```python
from build123d import *

# Parameters (mm, degrees)
SKETCH1_W           = 55.65
SKETCH1_H           = 70.9
BOSS_EXTRUDE1_DEPTH = 5
SKETCH3_W           = 53.15
SKETCH3_H           = 68.4
CUT_EXTRUDE1_DEPTH  = 3
SKETCH2_R           = 2.5
CUT_EXTRUDE2_DEPTH  = 6


with BuildPart() as part:
    # Sketch1 → Boss-Extrude1 (new body)
    with BuildSketch(Plane.XY):
        Rectangle(SKETCH1_W, SKETCH1_H)
    extrude(amount=BOSS_EXTRUDE1_DEPTH)

    # Sketch3 → Cut-Extrude1 (cut)
    with BuildSketch(Plane(origin=(0, 0, 0), x_dir=(-1, 0, 0), z_dir=(0, 0, -1))):
        Rectangle(SKETCH3_W, SKETCH3_H)
    extrude(amount=-CUT_EXTRUDE1_DEPTH, mode=Mode.SUBTRACT)

    # Sketch2 → Cut-Extrude2 (cut, through all)
    with BuildSketch(Plane(origin=(0, 0, 0), x_dir=(-1, 0, 0), z_dir=(0, 0, -1))):
        with Locations((-8.973470341, 31.308167243)):
            Circle(SKETCH2_R)
        with Locations((-23.973470341, -18.491832757)):
            Circle(SKETCH2_R)
        with Locations((23.676529659, -20.991832757)):
            Circle(SKETCH2_R)
        with Locations((19.676529659, 31.308167243)):
            Circle(SKETCH2_R)
    extrude(amount=-CUT_EXTRUDE2_DEPTH, mode=Mode.SUBTRACT)


solid = part.part
```
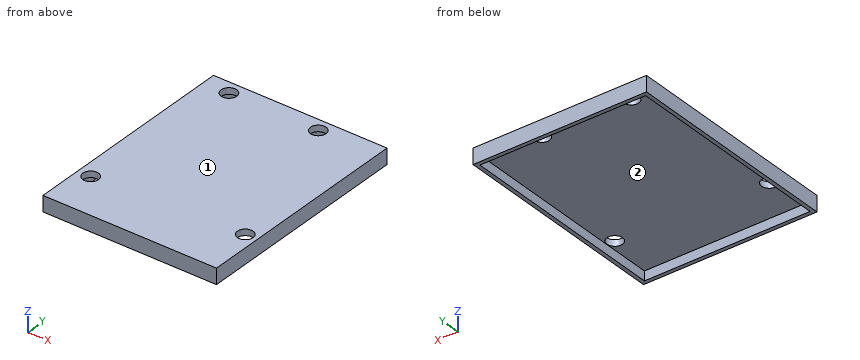
Verification items for the finished model (mm, model axes). Face numbers are marked on the shaded views. Round coordinates to 2 decimals unless told otherwise and drop trailing zeros. Write each loop counter-clockwise with the first axis right and the second up, starting at its lowest first coordinate (ties: lowest second). Pieces come first, ordered by that corner, then holes.
1. Section check D-D on x = -7.5. Enter the section's corners in (y, z).
2. Scan lines: L1, parallel to X at y = 3, z = 2.9 (3 decimals); L2, parallel to Y at x = 10, z = 1.25; L3, parallel to Y at x = 9, z = 3.4. Record each from-to range of solid material in increasing order.
3. Draft check along X on the marked faces 1 and 2. Enter one of: +X half, -X half, draft (parallel to the pull), parting line (faces both ways), or undercut.
4. Section check C-C on x = 9. Enter the section's corners in (y, z), plus the area to 3 significant figures.
5. Section check A-A on z = 1.9. Enter the section's corners in (x, y) (3 decimals).
6. Section check B-B on y = -2.5. Enter the section's corners in (x, z) (3 decimals).
7. Gauge pin test, flat end, axial feed: P1, Ø1.5, axis at x = 20.5, y = 8, coming from the -Z side. Record the tip position at first contact, or that the pin passes through.
Answer:
1. outline: (-35.45, 0) - (-34.2, 0) - (-34.2, 3) - (34.2, 3) - (34.2, 0) - (35.45, 0) - (35.45, 5) - (-35.45, 5) - close
2. L1: x = -27.825 to -26.575, 26.575 to 27.825
2. L2: y = -35.45 to -34.2, 34.2 to 35.45
2. L3: y = -35.45 to 28.81, 33.81 to 35.45
3. face 1: draft
3. face 2: undercut
4. outline: (-35.45, 0) - (-34.2, 0) - (-34.2, 3) - (28.81, 3) - (28.81, 5) - (-35.45, 5) - close; (33.81, 3) - (34.2, 3) - (34.2, 0) - (35.45, 0) - (35.45, 5) - (33.81, 5) - close
4. area: 139 mm2
5. outline: (-27.825, -35.45) - (27.825, -35.45) - (27.825, 35.45) - (-27.825, 35.45) - close; hole (-26.575, -34.2) - (26.575, -34.2) - (26.575, 34.2) - (-26.575, 34.2) - close
6. outline: (-27.825, 0) - (-26.575, 0) - (-26.575, 3) - (26.575, 3) - (26.575, 0) - (27.825, 0) - (27.825, 5) - (-27.825, 5) - close
7. P1: stops at z = 3
